Read the model definition and answer for the solid it produces. Units are mm, in the model's axes. A direction names the side the tool comes from. Coordinates: 2 decimals unless noted, no trailing zeros. Write each loop counter-clockwise with the first axis right and the second up, starting at its lowest first coordinate (ties: lowest second). Pieces come first, ordered by that corner, then holes.
Item 1: Section A-A (y = 8.89) is taken. Give the vertices of the cut face in (x, z).
Item 2: Straight lines are drawn through the part: probe 1 along Y at (x, z) = (0.25, 8.75); probe 2 along Y at (x, z) = (6.75, 1.5); probe 3 along Z at (x, y) = (2.5, -2.5). For each, find the intervals that lie inside material, in ascending order.
Item 3: Section C-C (z = 11.5) is taken. Give the vertices of the cut face in (x, y), then the cut area to 3 significant figures.
Item 4: Section B-B (x = 11.5) is taken. Give the vertices of the cut face in (y, z), then the cut area to 3 significant figures.
Item 5: Section D-D (x = 3.25) is taken. Give the vertices of the cut face in (y, z).
Item 6: Each of these flat-tipped pins is pushed along its axis until it touches: P1, Ø3, axis at y = 17, z = 1, coming from the +X side; P2, Ø6, axis at x = -1, y = 44, coming from the -Z side; P3, Ø5, axis at y = 15.5, z = 3.5, coming from the -X side. Where does it stop, or does it pass through?
Item 7: A tool of negligible diameter and unlimited length cuts with its end or side. For faces 1 (the face through (6.664, 23.8, 2.4)), 2 (the face through (0.33, 6.37, 9.79)), 3 (the face through (3.805, -3.757, 0.03)), 4 (the face through (-0.12, 52.02, 1.39)), from which of +Z, -Z, +X, -X, +Y, -Y can it reach the whole face along a straight path? Write none if from no direction.
Item 8: Determine the mould class of faces 5 (the face through (10.4, 8.1, 2.1)), 6 (the face through (0, 24, 0)), 7 (the face through (5.05, 48.26, 2.01)) for opening direction Y: released by +Y, released by -Y, zero draft, split by the parting line, or undercut.
from build123d import *

# Parameters (mm, degrees)
BOSS_EXTRUDE1_DEPTH = 48.26
SKETCH6_R           = 2.54
BOSS_EXTRUDE3_DEPTH = 7.62
SKETCH7_R           = 2.54
BOSS_EXTRUDE4_DEPTH = 7.62
SKETCH8_R           = 2.54
BOSS_EXTRUDE5_DEPTH = 7.62
SKETCH9_R           = 2.54
BOSS_EXTRUDE6_DEPTH = 7.62


with BuildPart() as part:
    # Sketch4 → Boss-Extrude1 (new body)
    with BuildSketch(Plane(origin=(0, 0, 0), x_dir=(1, 0, 0), z_dir=(0, 1, 0))):
        Polygon((-6.035613044, -6.035613044), (6.664386956, 6.664386956), (6.664386956, -6.035613044), align=None)
    extrude(amount=BOSS_EXTRUDE1_DEPTH)

    # Sketch6 → Boss-Extrude3 (add)
    with BuildSketch(Plane.XY.offset(6.035613044)):
        with Locations(Location((0, 8.89, 0), (0, 0, 180))):
            Circle(SKETCH6_R)
        with Locations(Location((0, 24.13, 0), (0, 0, 180))):
            Circle(SKETCH6_R)
        with Locations(Location((0, 39.37, 0), (0, 0, 180))):
            Circle(SKETCH6_R)
    extrude(amount=BOSS_EXTRUDE3_DEPTH)

    # Sketch7 → Boss-Extrude4 (add)
    with BuildSketch(Plane(origin=(6.664386956, 0, 0), x_dir=(0, 0, -1), z_dir=(1, 0, 0))):
        with Locations(Location((0.314386956, 8.89, 0), (0, 0, 180))):
            Circle(SKETCH7_R)
        with Locations(Location((0.314386956, 24.13, 0), (0, 0, 180))):
            Circle(SKETCH7_R)
        with Locations(Location((0.314386956, 39.37, 0), (0, 0, 180))):
            Circle(SKETCH7_R)
    extrude(amount=BOSS_EXTRUDE4_DEPTH)

    # Sketch8 → Boss-Extrude5 (add)
    with BuildSketch(Plane.XZ):
        with Locations(Location((2.25920074, 2.046048879, 0), (0, 0, 90))):
            Circle(SKETCH8_R)
    extrude(amount=BOSS_EXTRUDE5_DEPTH)

    # Sketch9 → Boss-Extrude6 (add)
    with BuildSketch(Plane(origin=(0, 48.26, 0), x_dir=(1, 0, 0), z_dir=(0, 1, 0))):
        with Locations(Location((2.360435834, -1.944813785, 0), (0, 0, 270))):
            Circle(SKETCH9_R)
    extrude(amount=BOSS_EXTRUDE6_DEPTH)


solid = part.part
Established:
1. outline: (-6.04, 6.04) - (6.66, -6.66) - (6.66, -2.85) - (14.28, -2.85) - (14.28, 2.23) - (6.66, 2.23) - (6.66, 6.04) - (2.54, 6.04) - (2.54, 13.66) - (-2.54, 13.66) - (-2.54, 6.04) - close
2. probe 1: y = 6.36 to 11.42, 21.6 to 26.66, 36.84 to 41.9
2. probe 2: y = 7.11 to 10.67, 22.35 to 25.91, 37.59 to 41.15
2. probe 3: z = -0.48 to 4.57
3. outline: circle Ø5.08 at (0, 8.89); circle Ø5.08 at (0, 24.13); circle Ø5.08 at (0, 39.37)
3. area: 60.8 mm2
4. outline: circle Ø5.08 at (8.89, -0.31); circle Ø5.08 at (24.13, -0.31); circle Ø5.08 at (39.37, -0.31)
4. area: 60.8 mm2
5. outline: (-7.62, -0.29) - (0, -0.29) - (0, -3.25) - (48.26, -3.25) - (48.26, -0.43) - (55.88, -0.43) - (55.88, 4.32) - (48.26, 4.32) - (48.26, 6.04) - (0, 6.04) - (0, 4.38) - (-7.62, 4.38) - close
6. P1: stops at x = 6.66
6. P2: stops at z = -2
6. P3: stops at x = -6
7. face 1: +X
7. face 2: +Z
7. face 3: -Y
7. face 4: +Y
8. face 5: undercut
8. face 6: zero draft
8. face 7: released by +Y
